Autodesk Inventor part; units mm, degrees
ref_plane "YZ Plane" through (0, 0, 0) normal (1, 0, 0) x (0, 1, 0)
ref_plane "XZ Plane" through (0, 0, 0) normal (0, 1, 0) x (-1, 0, 0)
ref_plane "XY Plane" through (0, 0, 0) normal (0, 0, 1) x (1, 0, 0)
sketch "Sketch1" plane through (0, 0, 0) normal (0, 0, 1) x (1, 0, 0)
  line L0 (32, 0) -> (32, -96)
  line L1 (-32, 0) -> (-32, -96)
  line L2 (32, 0) -> (-32, 0)
  line L3 (-32, 0) -> (-32, -96)
  line L4 (-32, -96) -> (32, -96)
  line L5 (32, -96) -> (32, 0)
  circle A0 centre (24, -16) radius 1.85
  circle A1 centre (16, -8) radius 1.85
  circle A2 centre (16, -16) radius 4
  circle A3 centre (16, -24) radius 1.85
  circle A4 centre (8, -16) radius 1.85
  circle A5 centre (16, -32) radius 4
  circle A6 centre (16, -40) radius 1.85
  circle A7 centre (16, -48) radius 4
  circle A8 centre (24, -48) radius 1.85
  circle A9 centre (16, -56) radius 1.85
  circle A10 centre (8, -48) radius 1.85
  circle A11 centre (16, -64) radius 4
  circle A12 centre (16, -72) radius 1.85
  circle A13 centre (24, -80) radius 1.85
  circle A14 centre (16, -88) radius 1.85
  circle A15 centre (8, -80) radius 1.85
  circle A16 centre (16, -80) radius 4
  circle A17 centre (-8, -80) radius 1.85
  circle A18 centre (-16, -80) radius 4
  circle A19 centre (-16, -72) radius 1.85
  circle A20 centre (-16, -88) radius 1.85
  circle A21 centre (-24, -80) radius 1.85
  circle A22 centre (-16, -64) radius 4
  circle A23 centre (-16, -56) radius 1.85
  circle A24 centre (-8, -48) radius 1.85
  circle A25 centre (-16, -40) radius 1.85
  circle A26 centre (-24, -48) radius 1.85
  circle A27 centre (-16, -48) radius 4
  circle A28 centre (-16, -32) radius 4
  circle A29 centre (-16, -24) radius 1.85
  circle A30 centre (-8, -16) radius 1.85
  circle A31 centre (-16, -8) radius 1.85
  circle A32 centre (-24, -16) radius 1.85
  circle A33 centre (-16, -16) radius 4
  point P0 (0, 0)
extrude "Extrusion1" add sketch "Sketch1" along normal blind 2
sketch "Sketch2" plane through (0, 0, 2) normal (0, 0, 1) x (1, 0, 0)
  circle A0 centre (24, -32) radius 1.85
  circle A1 centre (8, -32) radius 1.85
  circle A2 centre (8, -64) radius 1.85
  circle A3 centre (24, -64) radius 1.85
  circle A4 centre (-8, -32) radius 1.85
  circle A5 centre (-24, -32) radius 1.85
  circle A6 centre (-8, -64) radius 1.85
  circle A7 centre (-24, -64) radius 1.85
  point P0 (0, 0)
extrude "Extrusion2" cut sketch "Sketch2" against normal through all
sketch "Sketch3" plane through (0, 0, 2) normal (0, 0, 1) x (1, 0, 0)
  circle A0 centre (0, -8) radius 1.85
  circle A1 centre (0, -24) radius 1.85
  circle A2 centre (0, -32) radius 4
  circle A3 centre (0, -40) radius 1.85
  circle A4 centre (0, -16) radius 4
  circle A5 centre (0, -48) radius 4
  circle A6 centre (0, -56) radius 1.85
  circle A7 centre (0, -64) radius 4
  circle A8 centre (0, -72) radius 1.85
  circle A9 centre (0, -80) radius 4
  circle A10 centre (0, -88) radius 1.85
  point P0 (0, 0)
extrude "Extrusion3" cut sketch "Sketch3" against normal through all
Source: CAD feature listing. Evaluate the final solid. Frame: model axes, mm. Give positions to 0.01 mm unless a question says otherwise; leave off trailing zeros. Loops run counter-clockwise (first coordinate to the right, second up) from the corner with the lowest first, then second, coordinate; pieces in that order, holes last. Notation, with made-up numbers: (64.5, -10) -> (113.5, -10) arc R19 ccw to (113.5, 19) -> close; hole circle Ø7 at (-28, -24). An arc over 180 degrees is marked (long way). Use a Markdown table: item, result. Add a question column.
(1) Section query B-B (y = -32). Count the separate pieces of the cut face and the enclosed holes in it, then the cut area to 3 significant figures.
(2) Ray query, line 1 (Y direction, x = 8, z = 1.55); line 2 (Y direction, x = 6.5, z = 1.85); line 3 (X direction, y = -82, z = 1.75). Return the intervals inside material, ascending.
(3) Pull-direction query (X, two-part tool) for faces 1 (the face through (-15.146, -54.359, 0.986)), 2 (the face through (0, 0, 1)); classes: +X half, -X half, draft (parallel to the pull), parting line (faces both ways), or undercut.
(4) Section query A-A (x = 24). Output: boundary loops of the cut face in (y, z).
(5) Section query D-D (x = -7.5). Output: boundary loops of the cut face in (y, z).
Checked values:
| question | item | result |
|---|---|---|
| 1 | separate pieces | 8 |
| 1 | enclosed holes | 0 |
| 1 | area | 50.4 mm^2 |
| 2 | line 1 | -96 to -81.85, -78.15 to -65.85, -62.15 to -49.85, -46.15 to -33.85, -30.15 to -17.85, -14.15 to 0 |
| 2 | line 2 | -96 to -81.08, -78.92 to -65.08, -62.92 to -49.08, -46.92 to -33.08, -30.92 to -17.08, -14.92 to 0 |
| 2 | line 3 | -32 to -19.46, -12.54 to -3.46, 3.46 to 12.54, 19.46 to 32 |
| 3 | face 1 | undercut |
| 3 | face 2 | draft |
| 4 | outline | (-96, 0) -> (-81.85, 0) -> (-81.85, 2) -> (-96, 2) -> close; (-78.15, 0) -> (-65.85, 0) -> (-65.85, 2) -> (-78.15, 2) -> close; (-62.15, 0) -> (-49.85, 0) -> (-49.85, 2) -> (-62.15, 2) -> close; (-46.15, 0) -> (-33.85, 0) -> (-33.85, 2) -> (-46.15, 2) -> close; (-30.15, 0) -> (-17.85, 0) -> (-17.85, 2) -> (-30.15, 2) -> close; (-14.15, 0) -> (0, 0) -> (0, 2) -> (-14.15, 2) -> close |
| 5 | outline | (-96, 0) -> (-81.78, 0) -> (-81.78, 2) -> (-96, 2) -> close; (-78.22, 0) -> (-65.78, 0) -> (-65.78, 2) -> (-78.22, 2) -> close; (-62.22, 0) -> (-49.78, 0) -> (-49.78, 2) -> (-62.22, 2) -> close; (-46.22, 0) -> (-33.78, 0) -> (-33.78, 2) -> (-46.22, 2) -> close; (-30.22, 0) -> (-17.78, 0) -> (-17.78, 2) -> (-30.22, 2) -> close; (-14.22, 0) -> (0, 0) -> (0, 2) -> (-14.22, 2) -> close |
